Input: part model. Units: mm. Frame: model coordinates. Give positions to 0.01 mm unless a question says otherwise; leave off trailing zeros. Write each loop counter-clockwise with the first axis right and the second up, starting at its lowest first coordinate (ties: lowest second). Pieces come first, ordered by that corner, then holes. Notation, with made-up numbers: (71.5, 46) - (100.5, 46) arc R31 cw to (100.5, 77) - close; hole circle Ø7 at (23, 84.25). An arc over 180 degrees is marked (long way). Answer as CSV lines item,"result".
```python
from build123d import *

# Parameters (mm, degrees)
SKETCH1_R           = 2.4892
BOSS_EXTRUDE1_DEPTH = 2.286


with BuildPart() as part:
    # Sketch1 → Boss-Extrude1 (new body)
    with BuildSketch(Plane.XY):
        with BuildLine():
            Line((-258.218407496, 188.842880428), (-220.118407496, 188.842880428))
            ThreePointArc((-220.118407496, 188.842880428), (-215.628279435, 186.983008489), (-213.768407496, 182.492880428))
            Line((-213.768407496, 182.492880428), (-213.768407496, 131.692880428))
            ThreePointArc((-213.768407496, 131.692880428), (-211.908535556, 127.202752368), (-207.418407496, 125.342880428))
            Line((-207.418407496, 125.342880428), (-162.968407496, 125.342880428))
            ThreePointArc((-162.968407496, 125.342880428), (-158.478279435, 123.483008489), (-156.618407496, 118.992880428))
            Line((-156.618407496, 118.992880428), (-156.618407496, 80.892880428))
            ThreePointArc((-156.618407496, 80.892880428), (-158.478279435, 76.402752368), (-162.968407496, 74.542880428))
            Line((-162.968407496, 74.542880428), (-302.668407496, 74.542880428))
            ThreePointArc((-302.668407496, 74.542880428), (-307.158535556, 76.402752368), (-309.018407496, 80.892880428))
            Line((-309.018407496, 80.892880428), (-309.018407496, 118.992880428))
            ThreePointArc((-309.018407496, 118.992880428), (-307.158535556, 123.483008489), (-302.668407496, 125.342880428))
            Line((-302.668407496, 125.342880428), (-270.918407496, 125.342880428))
            ThreePointArc((-270.918407496, 125.342880428), (-266.428279435, 127.202752368), (-264.568407496, 131.692880428))
            Line((-264.568407496, 131.692880428), (-264.568407496, 182.492880428))
            ThreePointArc((-264.568407496, 182.492880428), (-262.708535556, 186.983008489), (-258.218407496, 188.842880428))
        make_face()
        with Locations((-226.468407496, 157.092880428)):
            Circle(SKETCH1_R, mode=Mode.SUBTRACT)
        with Locations((-226.468407496, 144.392880428)):
            Circle(SKETCH1_R, mode=Mode.SUBTRACT)
        with Locations((-226.468407496, 131.692880428)):
            Circle(SKETCH1_R, mode=Mode.SUBTRACT)
        with Locations((-239.168407496, 131.692880428)):
            Circle(SKETCH1_R, mode=Mode.SUBTRACT)
        with Locations((-251.868407496, 131.692880428)):
            Circle(SKETCH1_R, mode=Mode.SUBTRACT)
        with Locations((-251.868407496, 144.392880428)):
            Circle(SKETCH1_R, mode=Mode.SUBTRACT)
        with Locations((-239.168407496, 144.392880428)):
            Circle(SKETCH1_R, mode=Mode.SUBTRACT)
        with Locations((-239.168407496, 157.092880428)):
            Circle(SKETCH1_R, mode=Mode.SUBTRACT)
        with Locations((-251.868407496, 157.092880428)):
            Circle(SKETCH1_R, mode=Mode.SUBTRACT)
        with Locations((-226.468407496, 169.792880428)):
            Circle(SKETCH1_R, mode=Mode.SUBTRACT)
        with Locations((-226.468407496, 182.492880428)):
            Circle(SKETCH1_R, mode=Mode.SUBTRACT)
        with Locations((-239.168407496, 182.492880428)):
            Circle(SKETCH1_R, mode=Mode.SUBTRACT)
        with Locations((-239.168407496, 169.792880428)):
            Circle(SKETCH1_R, mode=Mode.SUBTRACT)
        with Locations((-251.868407496, 169.792880428)):
            Circle(SKETCH1_R, mode=Mode.SUBTRACT)
        with Locations((-251.868407496, 182.492880428)):
            Circle(SKETCH1_R, mode=Mode.SUBTRACT)
        with Locations((-302.668407496, 112.642880428)):
            Circle(SKETCH1_R, mode=Mode.SUBTRACT)
        with Locations((-289.968407496, 112.642880428)):
            Circle(SKETCH1_R, mode=Mode.SUBTRACT)
        with Locations((-277.268407496, 112.642880428)):
            Circle(SKETCH1_R, mode=Mode.SUBTRACT)
        with Locations((-264.568407496, 112.642880428)):
            Circle(SKETCH1_R, mode=Mode.SUBTRACT)
        with Locations((-251.868407496, 112.642880428)):
            Circle(SKETCH1_R, mode=Mode.SUBTRACT)
        with Locations((-239.168407496, 112.642880428)):
            Circle(SKETCH1_R, mode=Mode.SUBTRACT)
        with Locations((-226.468407496, 112.642880428)):
            Circle(SKETCH1_R, mode=Mode.SUBTRACT)
        with Locations((-213.768407496, 112.642880428)):
            Circle(SKETCH1_R, mode=Mode.SUBTRACT)
        with Locations((-201.068407496, 112.642880428)):
            Circle(SKETCH1_R, mode=Mode.SUBTRACT)
        with Locations((-188.368407496, 112.642880428)):
            Circle(SKETCH1_R, mode=Mode.SUBTRACT)
        with Locations((-175.668407496, 112.642880428)):
            Circle(SKETCH1_R, mode=Mode.SUBTRACT)
        with Locations((-162.968407496, 112.642880428)):
            Circle(SKETCH1_R, mode=Mode.SUBTRACT)
        with Locations((-289.968407496, 99.942880428)):
            Circle(SKETCH1_R, mode=Mode.SUBTRACT)
        with Locations((-277.268407496, 99.942880428)):
            Circle(SKETCH1_R, mode=Mode.SUBTRACT)
        with Locations((-264.568407496, 99.942880428)):
            Circle(SKETCH1_R, mode=Mode.SUBTRACT)
        with Locations((-251.868407496, 99.942880428)):
            Circle(SKETCH1_R, mode=Mode.SUBTRACT)
        with Locations((-239.168407496, 99.942880428)):
            Circle(SKETCH1_R, mode=Mode.SUBTRACT)
        with Locations((-226.468407496, 99.942880428)):
            Circle(SKETCH1_R, mode=Mode.SUBTRACT)
        with Locations((-213.768407496, 99.942880428)):
            Circle(SKETCH1_R, mode=Mode.SUBTRACT)
        with Locations((-201.068407496, 99.942880428)):
            Circle(SKETCH1_R, mode=Mode.SUBTRACT)
        with Locations((-188.368407496, 99.942880428)):
            Circle(SKETCH1_R, mode=Mode.SUBTRACT)
        with Locations((-175.668407496, 99.942880428)):
            Circle(SKETCH1_R, mode=Mode.SUBTRACT)
        with Locations((-162.968407496, 99.942880428)):
            Circle(SKETCH1_R, mode=Mode.SUBTRACT)
        with Locations((-289.968407496, 87.242880428)):
            Circle(SKETCH1_R, mode=Mode.SUBTRACT)
        with Locations((-277.268407496, 87.242880428)):
            Circle(SKETCH1_R, mode=Mode.SUBTRACT)
        with Locations((-264.568407496, 87.242880428)):
            Circle(SKETCH1_R, mode=Mode.SUBTRACT)
        with Locations((-251.868407496, 87.242880428)):
            Circle(SKETCH1_R, mode=Mode.SUBTRACT)
        with Locations((-239.168407496, 87.242880428)):
            Circle(SKETCH1_R, mode=Mode.SUBTRACT)
        with Locations((-226.468407496, 87.242880428)):
            Circle(SKETCH1_R, mode=Mode.SUBTRACT)
        with Locations((-213.768407496, 87.242880428)):
            Circle(SKETCH1_R, mode=Mode.SUBTRACT)
        with Locations((-201.068407496, 87.242880428)):
            Circle(SKETCH1_R, mode=Mode.SUBTRACT)
        with Locations((-188.368407496, 87.242880428)):
            Circle(SKETCH1_R, mode=Mode.SUBTRACT)
        with Locations((-175.668407496, 87.242880428)):
            Circle(SKETCH1_R, mode=Mode.SUBTRACT)
        with Locations((-162.968407496, 87.242880428)):
            Circle(SKETCH1_R, mode=Mode.SUBTRACT)
        with Locations((-302.668407496, 99.942880428)):
            Circle(SKETCH1_R, mode=Mode.SUBTRACT)
        with Locations((-302.668407496, 87.242880428)):
            Circle(SKETCH1_R, mode=Mode.SUBTRACT)
    extrude(amount=BOSS_EXTRUDE1_DEPTH)


solid = part.part
```
Item 1: Cut plane D-D on z = 0.9. Count the separate pieces of the cut face and the enclosed holes in it, plus the area to 3 significant figures.
The answers:
separate pieces,"1"
enclosed holes,"51"
area,"9,940 mm²"
Item 2: Contact query for a flat-ended pin moving along its axis: pin 1 (5 mm diameter, centred on x = -219, y = 122.5, fed in from -Z). Output: stop coordinate, or through.
The answers:
pin 1,"z = 0"
Item 3: Ray query, line 1 (Y direction, x = -302.5, z = 1.7); line 2 (Y direction, x = -214.5, z = 1.35); line 3 (X direction, y = 172, z = 2.25). Return the intervals inside material, ascending. Write a range as from..to.
The answers:
line 1,"74.54..84.76, 89.73..97.46, 102.43..110.16, 115.13..125.34"
line 2,"74.54..84.86, 89.62..97.56, 102.32..110.26, 115.02..185.45"
line 3,"-264.57..-253.02, -250.72..-240.32, -238.02..-227.62, -225.32..-213.77"
Item 4: Mould query, pull axis Y, two halves, no side actions, for faces 1 (the face through (-232, 120, 2.286)), 2 (the face through (-262.27, 86.29, 1.13)), 3 (the face through (-158.528, 123.532, 1.127)), 4 (the face through (-198.694, 113.391, 1.127)). Classes: +Y half, -Y half, draft (parallel to the pull), parting line (faces both ways), or undercut.
The answers:
face 1,"draft"
face 2,"undercut"
face 3,"+Y half"
face 4,"undercut"
Item 5: Cut plane C-C on y = 176. Return the cut outline in (x, z).
The answers:
outline,"(-264.57, 0) - (-213.77, 0) - (-213.77, 2.29) - (-264.57, 2.29) - close"
Item 6: Cut plane B-B on x = -175. Return the cut outline in (y, z), plus the area to 3 significant figures.
The answers:
outline,"(74.54, 0) - (84.85, 0) - (84.85, 2.29) - (74.54, 2.29) - close; (89.64, 0) - (97.55, 0) - (97.55, 2.29) - (89.64, 2.29) - close; (102.34, 0) - (110.25, 0) - (110.25, 2.29) - (102.34, 2.29) - close; (115.04, 0) - (125.34, 0) - (125.34, 2.29) - (115.04, 2.29) - close"
area,"83.2 mm²"
Item 7: Cut plane A-A on x = -290. Return the cut outline in (y, z).
The answers:
outline,"(74.54, 0) - (84.75, 0) - (84.75, 2.29) - (74.54, 2.29) - close; (89.73, 0) - (97.45, 0) - (97.45, 2.29) - (89.73, 2.29) - close; (102.43, 0) - (110.15, 0) - (110.15, 2.29) - (102.43, 2.29) - close; (115.13, 0) - (125.34, 0) - (125.34, 2.29) - (115.13, 2.29) - close"
